Could you check a few things on this model? Use its own coordinates, in mm. Round coordinates to 2 decimals unless told otherwise and drop trailing zeros. Order: outer loops, then holes, each group sorted by start corner. A loop starts at its lowest first (then second) coordinate and runs counter-clockwise, first axis right, second up. Notation, with made-up numbers: (33.25, 21.5) -> (41.25, 21.5) arc R19 cw to (41.25, 29.5) -> close; hole circle Ø11 at (49.5, 6). An arc over 180 degrees is marked (long way). One line per question, with ' | ' between items.
```python
from build123d import *

# Parameters (mm, degrees)
SKETCH1_R           = 4.7625
BOSS_EXTRUDE1_DEPTH = 5.5372


with BuildPart() as part:
    # Sketch1 → Boss-Extrude1 (new body)
    with BuildSketch(Plane.XY):
        Circle(SKETCH1_R)
        with BuildLine():
            Line((-2.667, 3.175), (2.667, 3.175))
            ThreePointArc((2.667, 3.175), (3.026210245, 3.026210245), (3.175, 2.667))
            Line((3.175, 2.667), (3.175, -2.667))
            ThreePointArc((3.175, -2.667), (3.026210245, -3.026210245), (2.667, -3.175))
            Line((2.667, -3.175), (-2.667, -3.175))
            ThreePointArc((-2.667, -3.175), (-3.026210245, -3.026210245), (-3.175, -2.667))
            Line((-3.175, -2.667), (-3.175, 2.667))
            ThreePointArc((-3.175, 2.667), (-3.026210245, 3.026210245), (-2.667, 3.175))
        make_face(mode=Mode.SUBTRACT)
    extrude(amount=BOSS_EXTRUDE1_DEPTH)


solid = part.part
```
1. I want a section at C-C on z = 2.6. List the corners of the cut face in (x, y) for me (1 decimal).
From the geometry:
outline: circle Ø9.5 at (0, 0); hole (-3.2, -2.7) arc R0.5 ccw to (-2.7, -3.2) -> (2.7, -3.2) arc R0.5 ccw to (3.2, -2.7) -> (3.2, 2.7) arc R0.5 ccw to (2.7, 3.2) -> (-2.7, 3.2) arc R0.5 ccw to (-3.2, 2.7) -> close
2. I want a section at D-D on y = 4.25. List the corners of the cut face in (x, z) for me.
From the geometry:
outline: (-2.15, 0) -> (2.15, 0) -> (2.15, 5.54) -> (-2.15, 5.54) -> close
3. If we mould it in two halves opening along X, with no side actions, what happens to faces 1 (the face through (0, 3.175, 3)), 2 (the face through (0, -3.175, 3)), 3 (the face through (-3.78, -2.9, 2.73))? For each: pulls with the +X half, pulls with the -X half, needs draft (parallel to the pull), parting line crosses it, or undercut.
From the geometry:
face 1: undercut | face 2: undercut | face 3: parting line crosses it
4. I need wall thicknesses on probe 1 along X at (y, z) = (-1.5, 3.6) (3 decimals); probe 2 along X at (y, z) = (-2.5, 3.7) (3 decimals); probe 3 along Y at (x, z) = (3, 4.3). Which ranges of each line are inside material? Lowest first, please.
From the geometry:
probe 1: x = -4.52 to -3.175, 3.175 to 4.52 | probe 2: x = -4.054 to -3.175, 3.175 to 4.054 | probe 3: y = -3.7 to -3.05, 3.05 to 3.7
5. I'm going to push flat-ended pins straight in: pin 1 (1.5 mm diameter, centred on x = 2, z = 1, fed in from -Y); pin 2 (1 mm diameter, centred on y = -2, z = 2.5, fed in from +X); pin 3 (1.5 mm diameter, centred on x = -3.5, z = 5, fed in from +Y). Where does each tip first touch, or does it pass through?
From the geometry:
pin 1: stops at y = -4.6 | pin 2: stops at x = 4.52 | pin 3: stops at y = 3.89
6. I want a section at A-A on x = 0. List the corners of the cut face in (y, z) for me (1 decimal), and give its area (3 significant figures).
From the geometry:
outline: (-4.8, 0) -> (-3.2, 0) -> (-3.2, 5.5) -> (-4.8, 5.5) -> close; (3.2, 0) -> (4.8, 0) -> (4.8, 5.5) -> (3.2, 5.5) -> close | area: 17.6 mm²
